from build123d import *

# Parameters (mm, degrees)
SKETCH1_R           = 24.6
BOSS_EXTRUDE1_DEPTH = 55
SKETCH2_R           = 4
BOSS_EXTRUDE2_DEPTH = 24.5
SKETCH3_W           = 19.796892184
SKETCH3_H           = 20
BOSS_EXTRUDE3_DEPTH = 5


with BuildPart() as part:
    # Sketch1 → Boss-Extrude1 (new body)
    with BuildSketch(Plane(origin=(0, 0, 0), x_dir=(1, 0, 0), z_dir=(0, 1, 0))):
        with Locations(Location((0, 0, 0), (0, 0, 270))):
            Circle(SKETCH1_R)
    extrude(amount=BOSS_EXTRUDE1_DEPTH)

    # Sketch2 → Boss-Extrude2 (add)
    with BuildSketch(Plane(origin=(0, 55, 0), x_dir=(1, 0, 0), z_dir=(0, 1, 0))):
        with Locations(Location((0, 0, 0), (0, 0, 270))):
            Circle(SKETCH2_R)
    extrude(amount=BOSS_EXTRUDE2_DEPTH)

    # Sketch3 → Boss-Extrude3 (add)
    with BuildSketch(Plane.XZ):
        with Locations((0, -32.520674168)):
            Rectangle(SKETCH3_W, SKETCH3_H)
    extrude(amount=-BOSS_EXTRUDE3_DEPTH)


solid = part.part
For this review, take the finished solid that the model builds, in its own axes (mm). A direction names the side the tool comes from. Coordinates: 2 decimals unless noted, no trailing zeros. Order: outer loops, then holes, each group sorted by start corner. A loop starts at its lowest first (then second) coordinate and runs counter-clockwise, first axis right, second up. Notation, with made-up numbers: (44, 50) - (81, 50) arc R14 cw to (81, 69) - close; hole circle Ø10 at (72, -8). An arc over 180 degrees is marked (long way). Answer as CSV lines item,"result". Start each with the question number.
1) Machinability: for faces 1 (the cylindrical face through (-3.905, 67.078, -0.867)), 2 (the flat face through (-9.898, 2, -33)), 3 (the flat face through (9.898, 2, -33)), which of the approach directions +Z, -Z, +X, -X, +Y, -Y give a long, thin tool a straight path to every point of the face, cutting with its end or side? Answer none if there is none.
2) Add section D-D (z = 13). State the section outline as (x, y) points, then the cut area to 3 significant figures.
3) Add section C-C (y = 71.5). State the section outline as (x, z) points.
4) Insertion check: P1, Ø1.5, axis at x = 10, z = -5, coming from the +Y side; P2, Ø8, axis at y = 56.5, z = 7.5, coming from the -X side; P3, Ø10, axis at x = 14, y = 63.5, coming from the +Z side; P4, Ø1.5, axis at y = 43.5, z = 17.5, coming from the +X side. Each pin has a flat end and moves straight along its axis. Give the tip position at first contact, or say it passes through.
5) Add section B-B (z = 0). State the section outline as (x, y) points.
6) Add section A-A (x = 0). State the section outline as (y, z) points.
7) To check wall thickness, follow line 1 along Y through (x, z) = (-17.5, 16.5); line 2 along X through (y, z) = (41, 6); line 3 along Z through (x, y) = (-12.5, 35.5). State the ranges of each line that lie inside material, in increasing order. Write a range as [from, to].
Result:
1,face 1,"+Y"
1,face 2,"-Z, -X, +Y, -Y"
1,face 3,"-Z, +X, +Y, -Y"
2,outline,"(-20.88, 0) - (20.88, 0) - (20.88, 55) - (-20.88, 55) - close"
2,area,"2,300 mm^2"
3,outline,"circle Ø8 at (0, 0)"
4,P1,"y = 55"
4,P2,"x = -24.31"
4,P3,"through"
4,P4,"x = 18.02"
5,outline,"(-24.6, 0) - (24.6, 0) - (24.6, 55) - (4, 55) - (4, 79.5) - (-4, 79.5) - (-4, 55) - (-24.6, 55) - close"
6,outline,"(0, -42.52) - (5, -42.52) - (5, -24.6) - (55, -24.6) - (55, -4) - (79.5, -4) - (79.5, 4) - (55, 4) - (55, 24.6) - (0, 24.6) - close"
7,line 1,"[0, 55]"
7,line 2,"[-23.86, 23.86]"
7,line 3,"[-21.19, 21.19]"
